Here's how the part is built. I have some questions about the finished solid (model axes, mm). Face numbers are marked on the shaded views. A direction names the side the tool comes from. Round coordinates to 2 decimals unless told otherwise and drop trailing zeros. Write each loop counter-clockwise with the first axis right and the second up, starting at its lowest first coordinate (ties: lowest second). Pieces come first, ordered by that corner, then holes. Notation, with made-up numbers: (-24.5, 18.25) - (9.5, 18.25) arc R32 cw to (9.5, 49.25) - close; hole circle Ø8 at (-14.75, 43.25). An arc over 180 degrees is marked (long way). Use one line per item in the form item = value. Start each with the question number.
1. I want a section at B-B, the plane z = -0.5. List the corners of the cut face in (x, y) for me.
2. Will these pins go through, and if not, where does the flat tip stop? pin 1 (1.6 mm diameter, centred on x = 18, y = 1, fed in from -Z); pin 2 (1.1 mm diameter, centred on x = 10.5, y = -0.5, fed in from +Z); pin 3 (1.1 mm diameter, centred on y = 0.5, z = -6, fed in from +X).
3. If I drill on line 1 along Z through (x, y) = (-1, 0.35); line 2 along X through (y, z) = (0.7, 2.5); line 3 along Z through (x, y) = (17.75, -0.8), over which ranges is the centre line in solid material (lowest first)?
4. I want a section at D-D, the plane z = 10.5. List the corners of the cut face in (x, y) for me.
5. I want a section at A-A, the plane x = 17.5. List the corners of the cut face in (y, z) for me, plus the area to 3 significant figures.
6. I want a section at C-C, the plane y = -0.3. List the corners of the cut face in (x, z) for me.
7. We'd pull the mould along X, two halves only. Please class the marked faces 1 and 2: +X half, -X half, draft (parallel to the pull), parting line (faces both ways), or undercut.
8. Which directions (+Z, -Z, +X, -X, +Y, -Y) give clear straight access to the entire face, cutting with the end or side of a thin tool? Please do the marked faces 3 and 4.
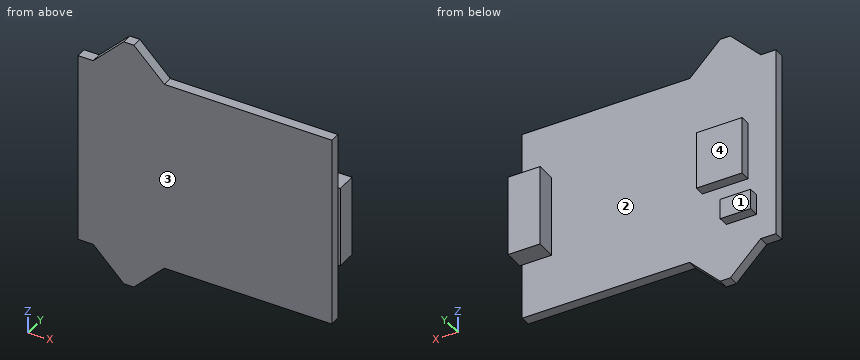
```python
from build123d import *

# Parameters (mm, degrees)
BOSS_EXTRUDE1_DEPTH = 1.000000032
SKETCH2_W           = 4.49999989
SKETCH2_H           = 5.735208424
SKETCH2_W_2         = 3
SKETCH2_H_2         = 2
BOSS_EXTRUDE2_DEPTH = 1
SKETCH3_W           = 3.154000042
SKETCH3_H           = 8.000000002
BOSS_EXTRUDE3_DEPTH = 1.94999991


with BuildPart() as part:
    # Sketch1 → Boss-Extrude1 (new body)
    with BuildSketch(Plane(origin=(0, 0, 0), x_dir=(1, 0, 0), z_dir=(0, 1, 0))):
        Polygon((-3.499999985, 9.50000005), (-0.499999889, 12.500000146), (0.499999889, 12.500000146), (3.499999985, 9.50000005), (4.999999906, 9.50000005), (20.000000132, 9.50000005), (20.000000132, -9.50000005), (4.999999906, -9.50000005), (3.499999985, -9.50000005), (0.499999889, -12.500000146), (-0.499999889, -12.500000146), (-3.499999985, -9.50000005), (-4.999999906, -9.50000005), (-4.999999906, 9.50000005), align=None)
    extrude(amount=-BOSS_EXTRUDE1_DEPTH)

    # Sketch2 → Boss-Extrude2 (add)
    with BuildSketch(Plane(origin=(0, 0, 0), x_dir=(1, 0, 0), z_dir=(0, 1, 0))):
        Rectangle(SKETCH2_W, SKETCH2_H)
        with Locations((-1.5875, 5.842)):
            Rectangle(SKETCH2_W_2, SKETCH2_H_2)
    extrude(amount=BOSS_EXTRUDE2_DEPTH)

    # Sketch3 → Boss-Extrude3 (add)
    with BuildSketch(Plane(origin=(0, 0, 0), x_dir=(1, 0, 0), z_dir=(0, 1, 0))):
        with Locations((18.677000111, 0)):
            Rectangle(SKETCH3_W, SKETCH3_H)
    extrude(amount=BOSS_EXTRUDE3_DEPTH)


solid = part.part
```
Model answer:
q1.outline = (-5, -1) - (20, -1) - (20, 0) - (20.25, 0) - (20.25, 1.95) - (17.1, 1.95) - (17.1, 0) - (2.25, 0) - (2.25, 1) - (-2.25, 1) - (-2.25, 0) - (-5, 0) - close
q2.pin_1 = -4
q2.pin_2 = 9.5
q2.pin_3 = 20
q3.line_1 = -6.84 to -4.84, -2.87 to 2.87
q3.line_2 = -2.25 to 2.25, 17.1 to 20.25
q3.line_3 = -9.5 to 9.5
q4.outline = (-2.5, -1) - (2.5, -1) - (2.5, 0) - (-2.5, 0) - close
q5.outline = (-1, -9.5) - (0, -9.5) - (0, -4) - (1.95, -4) - (1.95, 4) - (0, 4) - (0, 9.5) - (-1, 9.5) - close
q5.area = 34.6 mm2
q6.outline = (-5, -9.5) - (-3.5, -9.5) - (-0.5, -12.5) - (0.5, -12.5) - (3.5, -9.5) - (20, -9.5) - (20, 9.5) - (3.5, 9.5) - (0.5, 12.5) - (-0.5, 12.5) - (-3.5, 9.5) - (-5, 9.5) - close
q7.face_1 = draft
q7.face_2 = undercut
q8.face_3 = +Z, -Z, +X, -X, -Y
q8.face_4 = +Z, -Z, -X, +Y
